```python
from build123d import *

# Parameters (mm, degrees)
SKETCH1_R           = 13.97
BOSS_EXTRUDE1_DEPTH = 3.175
SKETCH2_W           = 3.175
SKETCH2_H           = 50.8
BOSS_EXTRUDE2_DEPTH = 40.64
FILLET1_R           = 1.5875
FILLET2_R           = 3.175
SKETCH6_R           = 3.175
CUT_EXTRUDE2_DEPTH  = 51.927
FILLET3_R           = 6.35


with BuildPart() as part:
    # Sketch1 → Boss-Extrude1 (new body)
    with BuildSketch(Plane(origin=(0, 0, 0), x_dir=(1, 0, 0), z_dir=(0, 1, 0))):
        with BuildLine():
            ThreePointArc((3.799431403, -18.926403172), (19.304, 0), (3.799431403, 18.926403172))
            Line((3.799431403, 18.926403172), (-28.448, 25.4))
            Line((-28.448, 25.4), (-31.623, 25.4))
            Line((-31.623, 25.4), (-31.623, -25.4))
            Line((-31.623, -25.4), (-28.448, -25.4))
            Line((-28.448, -25.4), (3.799431403, -18.926403172))
        make_face()
        Circle(SKETCH1_R, mode=Mode.SUBTRACT)
    extrude(amount=BOSS_EXTRUDE1_DEPTH)

    # Sketch2 → Boss-Extrude2 (add)
    with BuildSketch(Plane(origin=(0, 3.175, 0), x_dir=(1, 0, 0), z_dir=(0, 1, 0))):
        with Locations((-30.0355, 0)):
            Rectangle(SKETCH2_W, SKETCH2_H)
    extrude(amount=BOSS_EXTRUDE2_DEPTH)

    # Fillet1
    fillet1_edges = [part.edges().sort_by_distance(p)[0] for p in [
        (-28.448, 3.175, 0),
    ]]
    fillet(fillet1_edges, radius=FILLET1_R)

    # Fillet2
    fillet2_edges = [part.edges().sort_by_distance(p)[0] for p in [
        (-31.623, 0, 0),
    ]]
    fillet(fillet2_edges, radius=FILLET2_R)

    # Sketch6 → Cut-Extrude2 (cut, through all)
    with BuildSketch(Plane.ZY.offset(31.623)):
        with Locations((-19.05, 15.875)):
            Circle(SKETCH6_R)
        with Locations((19.05, 15.875)):
            Circle(SKETCH6_R)
    extrude(amount=-CUT_EXTRUDE2_DEPTH, mode=Mode.SUBTRACT)

    # Fillet3
    fillet3_edges = [part.edges().sort_by_distance(p)[0] for p in [
        (-30.0355, 43.815, -25.4),
        (-30.0355, 43.815, 25.4),
    ]]
    fillet(fillet3_edges, radius=FILLET3_R)


solid = part.part
```
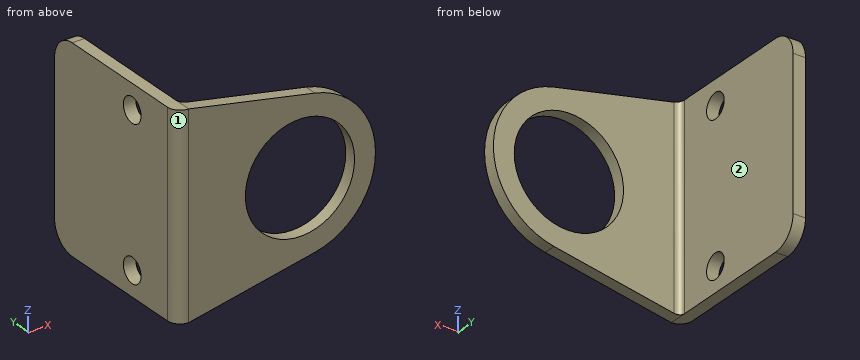
Input: part model. Units: mm. Frame: model coordinates. Face numbers are marked on the shaded views. A direction names the side the tool comes from. Give positions to 0.01 mm unless a question says otherwise; leave off trailing zeros. Order: outer loops, then holes, each group sorted by start corner. A loop starts at its lowest first (then second) coordinate and runs counter-clockwise, first axis right, second up. Notation, with made-up numbers: (68.5, -5.75) - (73.5, -5.75) arc R21 ccw to (73.5, 26.25) - close; hole circle Ø3 at (32.25, -20.5). An arc over 180 degrees is marked (long way). One line per item, written item: value.
1. Cut plane C-C, the plane y = 21.5. Output: boundary loops of the cut face in (x, z).
Determined:
outline: (-31.62, -25.4) - (-28.45, -25.4) - (-28.45, 25.4) - (-31.62, 25.4) - close
2. Line query: probe 1 along Y at (x, z) = (-25, -7) (3 decimals); probe 2 along X at (y, z) = (7.5, -3.5); probe 3 along Y at (x, z) = (-30.5, -19.05) (3 decimals). Output: solid intervals per line, ascending.
Determined:
probe 1: 0 to 3.175
probe 2: -31.62 to -28.45
probe 3: 0.752 to 12.7, 19.05 to 43.815
3. Reachability of the marked faces 1 and 2 from +Z, -Z, +X, -X, +Y, -Y: full face, straight path, thin tool, end or side. Return the list, or none.
Determined:
face 1: +Z, -Z, -X, -Y
face 2: +Z, -Z, +X, +Y
4. Pin query (flat end, axial travel): pin 1 Ø10 at (x, z) = (-10.5, 4.5) entering from -Y; pin 2 Ø2 at (x, z) = (9, -6.5) entering from -Y; pin 3 Ø11.5 at (y, z) = (25, 12) entering from +X; pin 4 Ø14 at (x, z) = (-5.5, -9) entering from +Y (3 decimals). Return the tip coordinate at first contact, or that it passes through.
Determined:
pin 1: y = 0
pin 2: through
pin 3: x = -28.45
pin 4: y = 3.175
5. Cut plane A-A, the plane x = 5. Output: boundary loops of the cut face in (y, z) (3 decimals), and give its area (3 significant figures).
Determined:
outline: (0, -18.645) - (3.175, -18.645) - (3.175, -13.045) - (0, -13.045) - close; (0, 13.045) - (3.175, 13.045) - (3.175, 18.645) - (0, 18.645) - close
area: 35.6 mm2
6. Cut plane D-D, the plane x = -2.5. Output: boundary loops of the cut face in (y, z) (3 decimals), and give its area (3 significant figures).
Determined:
outline: (0, -20.191) - (3.175, -20.191) - (3.175, -13.744) - (0, -13.744) - close; (0, 13.744) - (3.175, 13.744) - (3.175, 20.191) - (0, 20.191) - close
area: 40.9 mm2
